Job drawing, mm, ordinate dimensions from the low corner. One solid piece. A direction names the side the tool comes from. Give positions to 0.01 mm unless a question says otherwise; leave off trailing zeros. Order: outer loops, then holes, each group sorted by start corner. A loop starts at its lowest first (then second) coordinate and runs counter-clockwise, first axis right, second up.
Item 1: Which spindle directions (+Z, -Z, +X, -X, +Y, -Y) get a long thin tool onto all of the face, cutting with end or side? Do the marked faces 4, 5, 6, 7 and 8. Say none if no direction does.
Item 2: Band-saw the part on D-D on x = 27.5. Give the cut face in (y, z), plus the area to 3 significant figures.
Item 3: Wall check: L1, parallel to X at y = 16.75, z = 30; L2, parallel to Y at x = 15, z = 1.95; L3, parallel to Y at x = 11.75, z = 0.8. Give the ranges that are in metal, low to high.
Item 4: Band-saw the part on C-C on z = 30.5. Give the cut face in (x, y).
Item 5: Band-saw the part on A-A on z = 35.5. Give the cut face in (x, y).
Item 6: Flat gauge pins, fed straight in: P1, Ø2, axis at x = 26.5, z = 22, coming from the +Y side; P2, Ø2, axis at x = 2, z = 14.5, coming from the -Y side; P3, Ø3, axis at y = 15, z = 30.5, coming from the +X side. Where does each tip first touch, or does it go through?
Item 7: Band-saw the part on B-B on y = 15. Count the separate pieces of the cut face and the enclosed holes in it.
Item 8: Two-plate mould, pull along X, no slides. Class the marked faces 1, 2 and 3: released by +X, released by -X, zero draft, split by the parting line, or undercut.
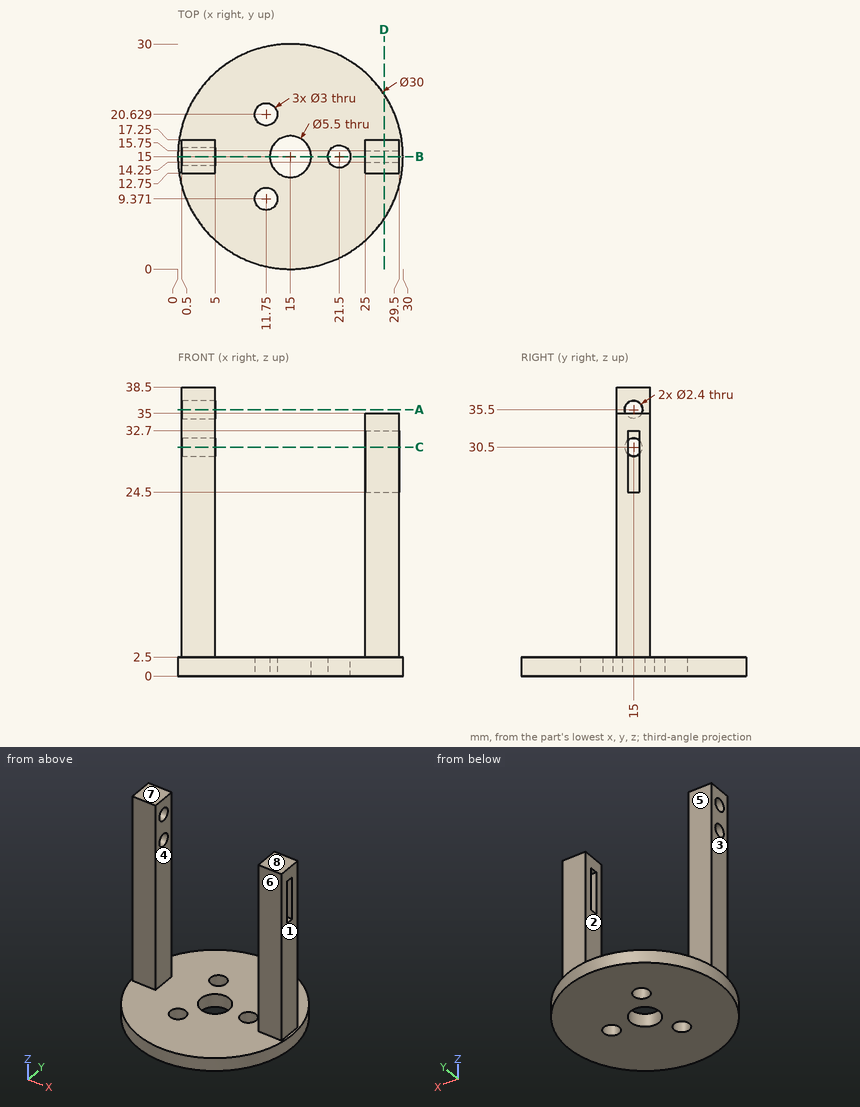
The answers:
1. face 4: +Z, +Y, -Y
1. face 5: +Z, +X, -X, +Y
1. face 6: +Z, +X, -X, -Y
1. face 7: +Z, +X, -X, +Y, -Y
1. face 8: +Z, +X, +Y, -Y
2. outline: (6.71, 0) - (23.29, 0) - (23.29, 2.5) - (17.25, 2.5) - (17.25, 35) - (12.75, 35) - (12.75, 2.5) - (6.71, 2.5) - close; hole (14.25, 24.5) - (15.75, 24.5) - (15.75, 32.7) - (14.25, 32.7) - close
2. area: 175 mm2
3. L1: x = 0.5 to 5, 25 to 29.5
3. L2: y = 0 to 12.25, 17.75 to 30
3. L3: y = 0.36 to 7.87, 10.87 to 19.13, 22.13 to 29.64
4. outline: (0.5, 12.75) - (5, 12.75) - (5, 13.8) - (0.5, 13.8) - close; (0.5, 16.2) - (5, 16.2) - (5, 17.25) - (0.5, 17.25) - close; (25, 12.75) - (29.5, 12.75) - (29.5, 14.25) - (25, 14.25) - close; (25, 15.75) - (29.5, 15.75) - (29.5, 17.25) - (25, 17.25) - close
5. outline: (0.5, 12.75) - (5, 12.75) - (5, 13.8) - (0.5, 13.8) - close; (0.5, 16.2) - (5, 16.2) - (5, 17.25) - (0.5, 17.25) - close
6. P1: stops at y = 17.25
6. P2: stops at y = 12.75
6. P3: stops at x = 29.5
7. separate pieces: 6
7. enclosed holes: 0
8. face 1: released by +X
8. face 2: undercut
8. face 3: released by -X
